```python
from build123d import *

# Parameters (mm, degrees)
F0_W     = 1.598067
F0_H     = 1.596714
F0_W_2   = 1.554564
F0_H_2   = 1.5875
F1_DEPTH = 30.999938


with BuildPart() as f1:
    # F0 (on Top) → F1 (new body)
    with BuildSketch(Plane.XY):
        Polygon((-1.21276, -1.837012), (-2.81296, -1.837012), (-2.81296, -3.424512), (-1.203091, -3.424512), (0.394976, -3.424512), (0.394976, -1.837012), (0.34934, -1.837012), align=None)
        Polygon((-1.21276, -0.229868), (-1.21276, -1.837012), (0.34934, -1.837012), (0.394976, -1.837012), (0.394976, -0.229868), align=None)
        with Locations((-0.404057, -4.222869)):
            Rectangle(F0_W, F0_H)
        with Locations((1.172258, -2.630762)):
            Rectangle(F0_W_2, F0_H_2)
    extrude(amount=F1_DEPTH)


solid = f1.part
```
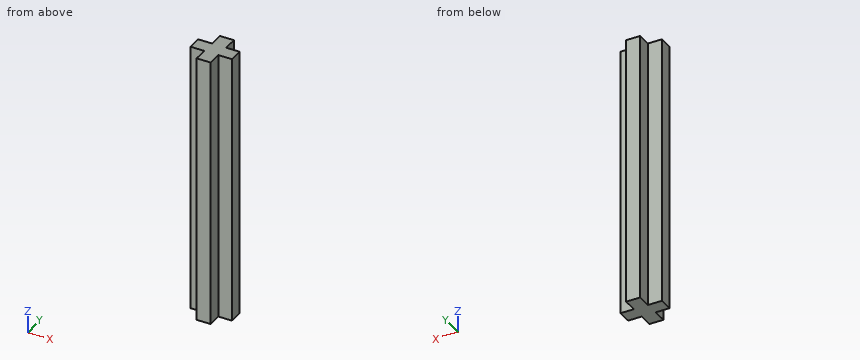
The listing builds one solid part. Answer for the finished solid, in the listing's coordinates (mm). Round coordinates to 2 decimals unless told otherwise and drop trailing zeros. Loops run counter-clockwise (first coordinate to the right, second up) from the corner with the lowest first, then second, coordinate; pieces in that order, holes last. Notation, with made-up numbers: (81.5, 57) -> (129.5, 57) arc R24 cw to (129.5, 94) -> close; hole circle Ø11 at (-16.75, 77.5). An arc over 180 degrees is marked (long way). Use one line per item in the form item = value.
1. The part is cut by section B-B on y = -1.2. Determine the outline of the cut face in (x, z).
Answer key:
outline = (-1.21, 0) -> (0.39, 0) -> (0.39, 31) -> (-1.21, 31) -> close
2. Flat-ended cylindrical pins translate along their axes: pin 1 Ø0.8 at (y, z) = (-1, 13.5) entering from -X; pin 2 Ø0.5 at (y, z) = (-0.5, 14.5) entering from +X (3 decimals); pin 3 Ø1.3 at (x, z) = (-2, 17.5) entering from +Y. Find the tip coordinate at first contact, or state that the pin passes through.
Answer key:
pin_1 = -1.21
pin_2 = 0.395
pin_3 = -1.84
3. Find the intervals of material crossed by probe 1 along Y at (x, z) = (-2.45, 11); probe 2 along X at (y, z) = (-4, 14.5), in increasing order. Write a range as [from, to].
Answer key:
probe_1 = [-3.42, -1.84]
probe_2 = [-1.2, 0.39]
4. The part is cut by section C-C on x = 1.15. Determine the outline of the cut face in (y, z), and give its area (3 significant figures).
Answer key:
outline = (-3.42, 0) -> (-1.84, 0) -> (-1.84, 31) -> (-3.42, 31) -> close
area = 49.2 mm²
5. The part is cut by section A-A on z = 6.5. Determine the outline of the cut face in (x, y), and give its area (3 significant figures).
Answer key:
outline = (-2.81, -3.42) -> (-1.2, -3.42) -> (-1.2, -5.02) -> (0.39, -5.02) -> (0.39, -3.42) -> (1.95, -3.42) -> (1.95, -1.84) -> (0.39, -1.84) -> (0.39, -0.23) -> (-1.21, -0.23) -> (-1.21, -1.84) -> (-2.81, -1.84) -> close
area = 12.7 mm²
